Can you work these out from the model? Positions are in its coordinate system, mm. Face numbers are marked on the shaded views. A direction names the side the tool comes from. Coordinates: 2 decimals unless noted, no trailing zeros. Loops run counter-clockwise (first coordinate to the right, second up) from the corner with the lowest first, then second, coordinate; pieces in that order, holes last.
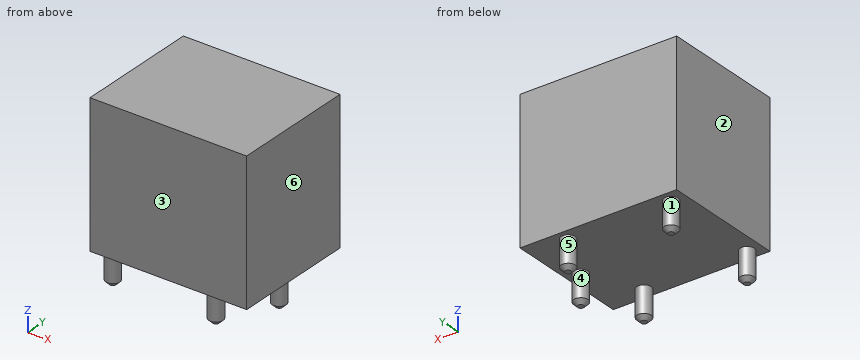
```python
from build123d import *

# Parameters (mm, degrees)
SKETCH1_W           = 15.5
SKETCH1_H           = 12.3
BOSS_EXTRUDE1_DEPTH = 7
SKETCH2_R           = 0.7
BOSS_EXTRUDE2_DEPTH = 3
CHAMFER1_SIZE       = 0.4


with BuildPart() as part:
    # Sketch1 → Boss-Extrude1 (new, symmetric)
    with BuildSketch(Plane.XY):
        Rectangle(SKETCH1_W, SKETCH1_H)
    extrude(amount=BOSS_EXTRUDE1_DEPTH, both=True)

    # Sketch2 → Boss-Extrude2 (add)
    with BuildSketch(Plane(origin=(0, 0, -7), x_dir=(-1, 0, 0), z_dir=(0, 0, -1))):
        with Locations(Location((-3.85, 5, 0), (0, 0, 180))):
            Circle(SKETCH2_R)
        with Locations(Location((6.35, 5, 0), (0, 0, 180))):
            Circle(SKETCH2_R)
        with Locations(Location((6.35, -5, 0), (0, 0, 180))):
            Circle(SKETCH2_R)
        with Locations(Location((-3.85, -5, 0), (0, 0, 180))):
            Circle(SKETCH2_R)
        with Locations(Location((-6.35, 0, 0), (0, 0, 180))):
            Circle(SKETCH2_R)
    extrude(amount=BOSS_EXTRUDE2_DEPTH)

    # Chamfer1
    chamfer1_edges = [part.edges().sort_by_distance(p)[0] for p in [
        (3.15, 5, -10),
        (-7.05, 5, -10),
        (-7.05, -5, -10),
        (3.15, -5, -10),
        (5.65, 0, -10),
    ]]
    chamfer(chamfer1_edges, length=CHAMFER1_SIZE)


solid = part.part
```
Item 1: I'm going to push a flat-ended pin straight in: P1, Ø6, axis at y = 1, z = -8, coming from the +X side. Where does the tip first touch, or does it pass through?
Results are:
P1: stops at x = 7.75
Item 2: On a 3-axis mill with a long thin cutter (end or side, diameter ignored), from which of +Z, -Z, +X, -X, +Y, -Y can I reach the whole of each face in a straight line? I mean the marked faces 5 and 6. Say none if no direction works.
Results are:
face 5: -Z
face 6: +Z, -Z, +X, +Y, -Y
Item 3: Suppose I cut it at C-C, the plane y = 5. Please give me the cut outline in (x, z).
Results are:
outline: (-7.75, -7) - (-7.05, -7) - (-7.05, -9.6) - (-6.65, -10) - (-6.05, -10) - (-5.65, -9.6) - (-5.65, -7) - (3.15, -7) - (3.15, -9.6) - (3.55, -10) - (4.15, -10) - (4.55, -9.6) - (4.55, -7) - (7.75, -7) - (7.75, 7) - (-7.75, 7) - close
Item 4: Suppose I cut it at B-B, the plane x = 6.35. Please give me the cut outline in (y, z).
Results are:
outline: (-6.15, -7) - (-0.7, -7) - (-0.7, -9.6) - (-0.3, -10) - (0.3, -10) - (0.7, -9.6) - (0.7, -7) - (6.15, -7) - (6.15, 7) - (-6.15, 7) - close
Item 5: We'd pull the mould along Y, two halves only. Please class the marked faces 1, 2, 3 and 4: +Y half, -Y half, draft (parallel to the pull), parting line (faces both ways), or undercut.
Results are:
face 1: undercut
face 2: draft
face 3: -Y half
face 4: parting line
Item 6: Suppose I cut it at A-A, the plane y = 0. Please give me the cut outline in (x, z).
Results are:
outline: (-7.75, -7) - (5.65, -7) - (5.65, -9.6) - (6.05, -10) - (6.65, -10) - (7.05, -9.6) - (7.05, -7) - (7.75, -7) - (7.75, 7) - (-7.75, 7) - close
Item 7: Suppose I cut it at D-D, the plane x = 3.85. Please give me the cut outline in (y, z), plus the area to 3 significant figures.
Results are:
outline: (-6.15, -7) - (-5.7, -7) - (-5.7, -9.6) - (-5.3, -10) - (-4.7, -10) - (-4.3, -9.6) - (-4.3, -7) - (4.3, -7) - (4.3, -9.6) - (4.7, -10) - (5.3, -10) - (5.7, -9.6) - (5.7, -7) - (6.15, -7) - (6.15, 7) - (-6.15, 7) - close
area: 180 mm2
Item 8: I need wall thicknesses on line 1 along Z through (x, y) = (-2.25, 3.5); line 2 along Z through (x, y) = (3.5, -4.75). Which ranges of each line are inside material? Lowest first, please.
Results are:
line 1: z = -7 to 7
line 2: z = -9.87 to 7
